Work out the finished part from the listing and answer in its coordinate system (mm). Face numbers are marked on the shaded views. A direction names the side the tool comes from. Round coordinates to 2 decimals unless told otherwise and drop trailing zeros. Write each loop counter-clockwise with the first axis right and the second up, starting at its lowest first coordinate (ties: lowest second). Pieces come first, ordered by that corner, then holes. Notation, with made-up numbers: M 37.5,33.25 L 68.5,33.25 A33 ccw 68.5,69.25 Z; hole C 44.5,13 d2. An arc over 180 degrees is marked long. Answer in a Markdown table with one row per item.
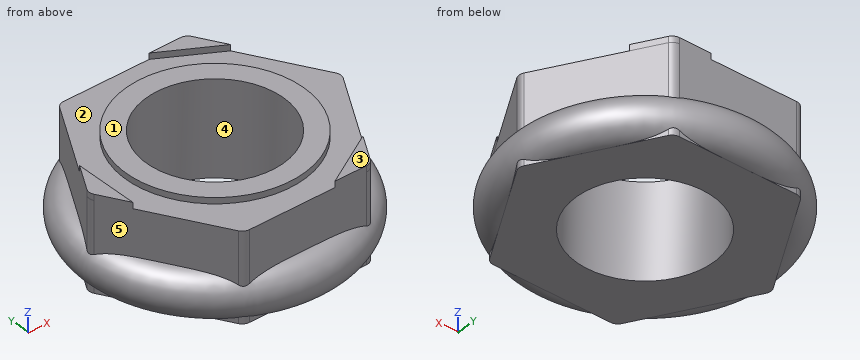
```python
from build123d import *

# Parameters (mm, degrees)
F0_R            = 4
F1_DEPTH        = 5.15
F2_R            = 0.5
F4_DEPTH        = 0.35
F4_COPIES_COUNT = 3
F3_R            = 5.2
F3_R_2          = 4
F5_DEPTH        = 0.35


# Not quite as in the source:
# - a pattern or mirror of a feature is missing from the dataset's text; its kind, count and spacing are read off the source's solid


with BuildPart() as f1:
    # F0 (on Top) → F1 (new body)
    with BuildSketch(Plane.XY):
        Polygon((3.75, 6.4951905284), (-3.75, 6.4951905284), (-7.5, 0), (-3.75, -6.4951905284), (3.75, -6.4951905284), (7.5, 0), align=None)
        Circle(F0_R, mode=Mode.SUBTRACT)
    extrude(amount=F1_DEPTH)

    # F2
    f2_edges = [f1.edges().sort_by_distance(p)[0] for p in [
        (3.75, -6.495191, 2.575),
        (7.5, 0, 2.575),
        (3.75, 6.495191, 2.575),
        (-3.75, 6.495191, 2.575),
        (-7.5, 0, 2.575),
        (-3.75, -6.495191, 2.575),
    ]]
    fillet(f2_edges, radius=F2_R)

    # F3 (on face) → F4 (join)
    with BuildSketch(Plane.XY.offset(5.15)):
        with BuildLine():
            Line((-6.4226497308, 1.8660254038), (-7.3556624327, 0.25))
            ThreePointArc((-7.3556624327, 0.25), (-7.4226497308, 0), (-7.3556624327, -0.25))
            Line((-7.3556624327, -0.25), (-6.4226497308, -1.8660254038))
            Line((-6.4226497308, -1.8660254038), (-6.4226497308, 1.8660254038))
        make_face()
    f4 = extrude(amount=F4_DEPTH)

    # F4_copies: F4 ×3 about axis
    f4_copies_axis = Axis((0, 0, 0), (0, 0, 1))
    for i in range(1, F4_COPIES_COUNT):
        add(f4.rotate(f4_copies_axis, i * 360 / F4_COPIES_COUNT))

    # F3 (on face) → F5 (join, through all)
    with BuildSketch(Plane.XY.offset(5.15)):
        Circle(F3_R)
        Circle(F3_R_2, mode=Mode.SUBTRACT)
    extrude(amount=F5_DEPTH)

    # F6 (on Right) → F7 (revolve)
    with BuildSketch(Plane.YZ):
        with BuildLine():
            ThreePointArc((-6.4951905284, 2.5), (-7.7451905284, 1.25), (-6.4951905284, 0))
            Line((-6.4951905284, 0), (-6.4951905284, 2.5))
        make_face()
    revolve(axis=Axis((0, 0, -0.6419573572), (0, 0, -1)))


solid = f1.part
```
1. A tool of negligible diameter and unlimited length cuts with its end or side. For the marked faces 1 and 2, from which of +Z, -Z, +X, -X, +Y, -Y can it reach the whole face along a straight path? Write none if from no direction.
Calculated:
| item | result |
|---|---|
| face 1 | +Z, +X, -X, +Y, -Y |
| face 2 | +Z |
2. Determine the mould class of the marked faces 3, 4 and 5 for opening direction X: released by +X, released by -X, zero draft, split by the parting line, or undercut.
Calculated:
| item | result |
|---|---|
| face 3 | zero draft |
| face 4 | undercut |
| face 5 | released by -X |
3. The part is cut by section B-B (z = 3.65). Determine the outline of the cut face in (x, y).
Calculated:
| item | result |
|---|---|
| outline | M -7.36,-0.25 L -3.89,-6.25 A0.5 ccw -3.46,-6.5 L 3.46,-6.5 A0.5 ccw 3.89,-6.25 L 7.36,-0.25 A0.5 ccw 7.36,0.25 L 3.89,6.25 A0.5 ccw 3.46,6.5 L -3.46,6.5 A0.5 ccw -3.89,6.25 L -7.36,0.25 A0.5 ccw Z; hole C 0,0 d8 |
4. The part is cut by section A-A (y = 0). Determine the outline of the cut face in (x, z).
Calculated:
| item | result |
|---|---|
| outline | M -7.42,0 L -4,0 L -4,5.5 L -5.2,5.5 L -5.2,5.15 L -6.42,5.15 L -6.42,5.5 L -7.42,5.5 L -7.42,2.09 A1.25 ccw -7.42,0.41 Z; M 4,0 L 7.42,0 L 7.42,0.41 A1.25 ccw 7.42,2.09 L 7.42,5.15 L 5.2,5.15 L 5.2,5.5 L 4,5.5 Z |
5. Given pin 1 (1 mm diameter, centred on x = 6, y = -3.5, fed in from +Z); pin 2 (2 mm diameter, centred on y = 2, z = 3, fed in from -X); pin 3 (2 mm diameter, centred on x = -4.5, z = 1.5, fed in from +Y), each flat-ended and moving along its own axis, determine where each tip first touches the part or whether it passes through.
Calculated:
| item | result |
|---|---|
| pin 1 | stops at z = 5.15 |
| pin 2 | stops at x = -7.26 |
| pin 3 | stops at y = 6.9 |
6. Consider line 1 along Y through (x, z) = (0, 4.35); line 2 along Z through (x, y) = (-4.5, 3.5); line 3 along Y through (x, z) = (-3.25, 1.95). Determine where each line is inside the solid, lowest interval first. Write a range as from..to.
Calculated:
| item | result |
|---|---|
| line 1 | y = -6.5..-4, 4..6.5 |
| line 2 | z = 0..5.15 |
| line 3 | y = -6.79..-2.33, 2.33..6.79 |
